Can you work these out from the drawing? Everything is in mm from the part's minimum corner. Coordinates: 2 decimals unless noted, no trailing zeros. Write each loop counter-clockwise with the first axis right and the second up, starting at its lowest first coordinate (ties: lowest second). Pieces come first, ordered by that corner, then holes.
(1) Imagine slicing it at B-B, the plane x = 12.25. List the corners of the cut face in (y, z) for me.
(2) Please list where these lines run through material, in increasing order: probe 1 along X at (y, z) = (0.75, 134.75); probe 2 along Z at (x, y) = (12.25, 0.65); probe 3 along Z at (x, y) = (16, 3.5).
(3) For pin 1 Ø1.5 at (y, z) = (3.5, 99) entering from -X; pin 2 Ø7 at (x, z) = (12.25, 134.75) entering from +Y; pin 3 Ø5 at (x, z) = (72.25, 14.75) entering from +Y, each with a flat end and sliding along its axis, tell me the tip position at first contact or that it passes through.
(4) Imagine slicing it at A-A, the plane z = 134.75. List the corners of the cut face in (x, y) for me, plus the area to 3 significant figures.
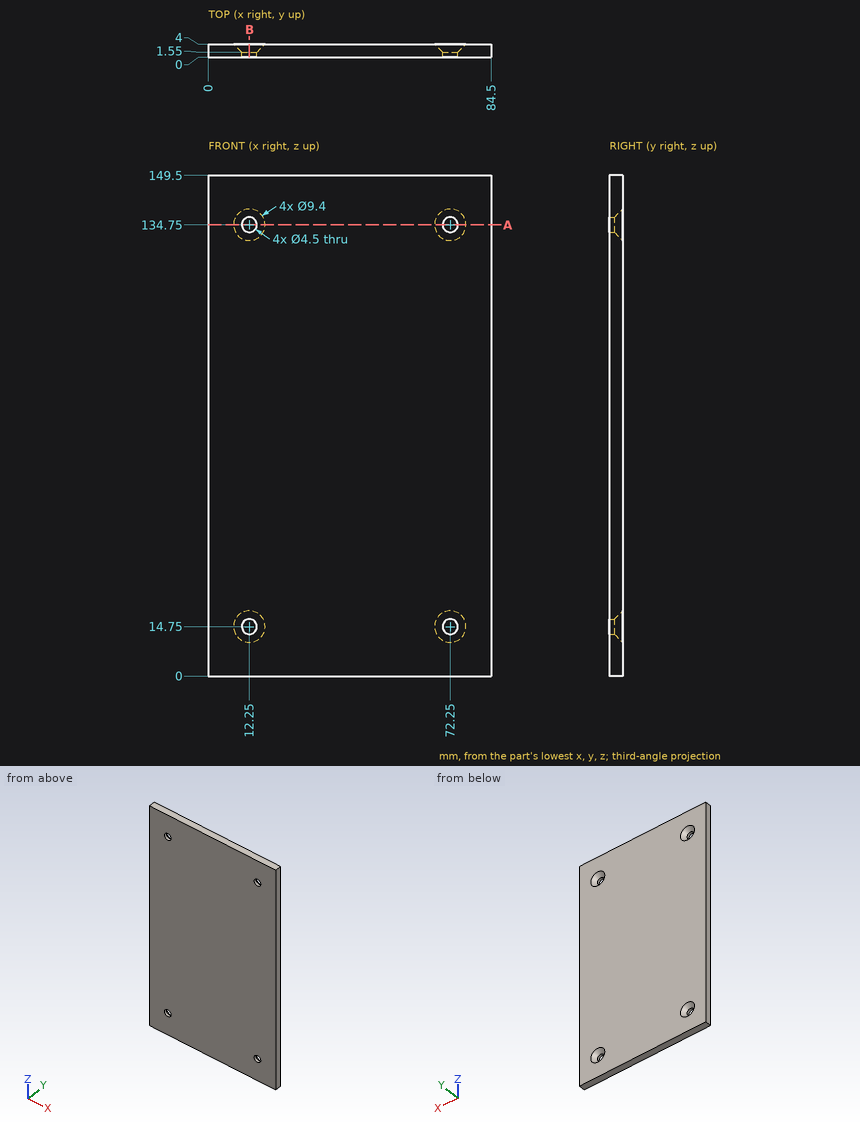
Recorded:
1. outline: (0, 0) - (4, 0) - (4, 10.05) - (1.55, 12.5) - (0, 12.5) - close; (0, 17) - (1.55, 17) - (4, 19.45) - (4, 130.05) - (1.55, 132.5) - (0, 132.5) - close; (0, 137) - (1.55, 137) - (4, 139.45) - (4, 149.5) - (0, 149.5) - close
2. probe 1: x = 0 to 10, 14.5 to 70, 74.5 to 84.5
2. probe 2: z = 0 to 12.5, 17 to 132.5, 137 to 149.5
2. probe 3: z = 0 to 12.86, 16.64 to 132.86, 136.64 to 149.5
3. pin 1: stops at x = 0
3. pin 2: stops at y = 2.8
3. pin 3: stops at y = 1.8
4. outline: (0, 0) - (10, 0) - (10, 1.55) - (7.55, 4) - (0, 4) - close; (14.5, 0) - (70, 0) - (70, 1.55) - (67.55, 4) - (16.95, 4) - (14.5, 1.55) - close; (74.5, 0) - (84.5, 0) - (84.5, 4) - (76.95, 4) - (74.5, 1.55) - close
4. area: 290 mm2
